Can you work these out from the model? Positions are in its coordinate system, mm. A direction names the side the tool comes from. Round coordinates to 2 decimals unless told otherwise and drop trailing zeros. Write each loop counter-clockwise with the first axis right and the second up, starting at its lowest first coordinate (ties: lowest second). Pieces come first, ordered by that corner, then holes. Notation, with made-up numbers: (23.25, -12.75) -> (63.25, -12.75) arc R29 cw to (63.25, 10.25) -> close; hole circle Ø8 at (4, -11.5). An arc over 180 degrees is marked (long way). Use CSV: the item, a comma, the result in double quotes.
```python
from build123d import *

# Parameters (mm, degrees)
SKETCH1_R           = 4
SKETCH1_R_2         = 2
BOSS_EXTRUDE1_DEPTH = 2


with BuildPart() as part:
    # Sketch1 → Boss-Extrude1 (new body)
    with BuildSketch(Plane(origin=(0, 0, 0), x_dir=(0, 0, -1), z_dir=(1, 0, 0))):
        with BuildLine():
            Line((121.29692104, -40.99299677), (121.29692104, -5.99299677))
            Line((121.29692104, -5.99299677), (86.29692104, -5.99299677))
            Line((86.29692104, -5.99299677), (86.29692104, -25.99299677))
            ThreePointArc((86.29692104, -25.99299677), (84.989984977, -32.116721127), (81.29692104, -37.173336658))
            Line((81.29692104, -37.173336658), (81.29692104, -40.99299677))
            Line((81.29692104, -40.99299677), (121.29692104, -40.99299677))
        make_face()
        with Locations((103.011400413, -23.49299677)):
            Circle(SKETCH1_R, mode=Mode.SUBTRACT)
        with Locations((116.011400413, -10.49299677)):
            Circle(SKETCH1_R_2, mode=Mode.SUBTRACT)
        with Locations((90.011400413, -36.49299677)):
            Circle(SKETCH1_R_2, mode=Mode.SUBTRACT)
    extrude(amount=BOSS_EXTRUDE1_DEPTH)


solid = part.part
```
Q1. Suppose I cut it at A-A (z = -101.5). Write out the boundary of the cut face in (x, y).
Resolved:
outline,"(0, -40.99) -> (2, -40.99) -> (2, -27.2) -> (0, -27.2) -> close; (0, -19.79) -> (2, -19.79) -> (2, -5.99) -> (0, -5.99) -> close"
Q2. Suppose I cut it at D-D (y = -13.5). Write out the boundary of the cut face in (x, z), and give its area (3 significant figures).
Resolved:
outline,"(0, -121.3) -> (2, -121.3) -> (2, -86.3) -> (0, -86.3) -> close"
area,"70.0 mm^2"
Q3. Suppose I cut it at C-C (x = 0.7). Write out the boundary of the cut face in (y, z).
Resolved:
outline,"(-40.99, -121.3) -> (-5.99, -121.3) -> (-5.99, -86.3) -> (-25.99, -86.3) arc R15 cw to (-37.17, -81.3) -> (-40.99, -81.3) -> close; hole circle Ø4 at (-36.49, -90.01); hole circle Ø8 at (-23.49, -103.01); hole circle Ø4 at (-10.49, -116.01)"
Q4. If we mould it in two halves opening along Y, with no side actions, what happens to faces 3 (the face through (1, -40.993, -101)), 4 (the face through (1, -39, -81.297)), 5 (the face through (0.986, -10.405, -114.013)), 6 (the face through (1, -5.993, -104))? For each: released by +Y, released by -Y, zero draft, split by the parting line, or undercut.
Resolved:
face 3,"released by -Y"
face 4,"zero draft"
face 5,"undercut"
face 6,"released by +Y"
Q5. Suppose I cut it at B-B (y = -36). Write out the boundary of the cut face in (x, z).
Resolved:
outline,"(0, -121.3) -> (2, -121.3) -> (2, -91.95) -> (0, -91.95) -> close; (0, -88.07) -> (2, -88.07) -> (2, -82.47) -> (0, -82.47) -> close"
Q6. Will these pins go through, and if not, where does the flat tip stop? P1, Ø7, axis at y = -23.49, z = -103.01, coming from the -X side; P2, Ø1, axis at x = 1, y = -12.5, coming from the +Z side.
Resolved:
P1,"passes through"
P2,"stops at z = -86.3"
Q7. On a 3-axis mill with a long thin cutter (end or side, diameter ignored), from which of +Z, -Z, +X, -X, +Y, -Y can I reach the whole of each face in a straight line? I mean faces 1 (the face through (1, -16, -86.297)), 2 (the face through (0.986, -25.025, -106.706)). Say none if no direction works.
Resolved:
face 1,"+Z, +X, -X, +Y"
face 2,"+X, -X"
Q8. Please list where these lines run through material, in increasing order: probe 1 along Z at (x, y) = (0.1, -8); probe 2 along Z at (x, y) = (0.3, -25.5); probe 3 along Y at (x, z) = (0.9, -104).
Resolved:
probe 1,"z = -121.3 to -86.3"
probe 2,"z = -121.3 to -106.47, -99.55 to -86.3"
probe 3,"y = -40.99 to -27.37, -19.62 to -5.99"
